The model under review builds one solid part; all positions refer to its coordinate system, in mm. Face numbers are marked on the shaded views. A direction names the side the tool comes from. Give positions to 0.01 mm unless a question says otherwise; leave off trailing zeros. Loops run counter-clockwise (first coordinate to the right, second up) from the corner with the lowest first, then second, coordinate; pieces in that order, holes last. Notation, with made-up numbers: M 11.5,86.25 L 54.5,86.25 A33 cw 54.5,125.25 Z; hole C 46.5,-26 d9. An arc over 180 degrees is marked long. Return JSON: item names as keys, results as strings. Group by question number.
```python
from build123d import *

# Parameters (mm, degrees)
EXTRUDE_1_DEPTH     = 35
EXTRUDE_2_DEPTH     = 3
SKETCH_3_R          = 4
CUT_EXTRUDE_1_DEPTH = 112.130553854
SKETCH_4_R          = 4
CUT_EXTRUDE_2_DEPTH = 112.130553854
FILLET_1_R          = 2
FILLET_2_R          = 2


with BuildPart() as part:
    # 草图1 → 凸台-拉伸1 (new body)
    with BuildSketch(Plane.XY):
        Polygon((0, 0), (78, 0), (78, 78), (71, 78), (71, 7), (0, 7), align=None)
    extrude(amount=EXTRUDE_1_DEPTH)

    # 草图2 → 凸台-拉伸2 (add)
    with BuildSketch(Plane(origin=(0, 0, 0), x_dir=(-1, 0, 0), z_dir=(0, 0, -1))):
        Polygon((-78, 78), (-78, 0), (0, 0), (0, 12.5), (-8, 12.5), (-65.5, 70), (-65.5, 78), align=None)
    extrude(amount=EXTRUDE_2_DEPTH)

    # 草图3 → 切除-拉伸1 (cut, through all)
    with BuildSketch(Plane.ZY.offset(-71)):
        with Locations((16, 58)):
            Circle(SKETCH_3_R)
        with BuildLine():
            Line((12, 41), (12, 23))
            ThreePointArc((12, 23), (16, 19), (20, 23))
            Line((20, 23), (20, 41))
            ThreePointArc((20, 41), (16, 45), (12, 41))
        make_face()
    extrude(amount=-CUT_EXTRUDE_1_DEPTH, mode=Mode.SUBTRACT)

    # 草图4 → 切除-拉伸2 (cut, through all)
    with BuildSketch(Plane(origin=(0, 7, 0), x_dir=(1, 0, 0), z_dir=(0, 1, 0))):
        with Locations(Location((20, -16, 0), (0, 0, 270))):
            Circle(SKETCH_4_R)
        with BuildLine():
            Line((37, -20), (55, -20))
            ThreePointArc((55, -20), (59, -16), (55, -12))
            Line((55, -12), (37, -12))
            ThreePointArc((37, -12), (33, -16), (37, -20))
        make_face()
    extrude(amount=-CUT_EXTRUDE_2_DEPTH, mode=Mode.SUBTRACT)

    # 圆角1
    fillet_1_edges = [part.edges().sort_by_distance(p)[0] for p in [
        (65.5, 78, -1.5),
        (0, 12.5, -1.5),
    ]]
    fillet(fillet_1_edges, radius=FILLET_1_R)

    # 圆角2
    fillet_2_edges = [part.edges().sort_by_distance(p)[0] for p in [
        (8, 12.5, -1.5),
        (65.5, 70, -1.5),
    ]]
    fillet(fillet_2_edges, radius=FILLET_2_R)


solid = part.part
```
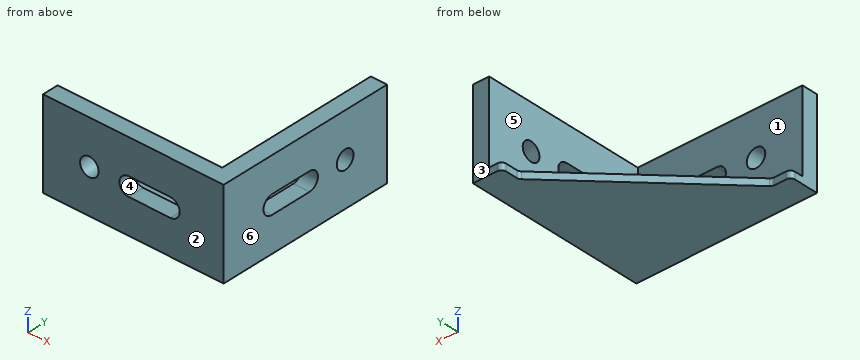
(1) For probe 1 along X at (y, z) = (4.25, 16); probe 2 along Y at (x, z) = (73.75, 16); probe 3 along Y at (x, z) = (62, 7), list the stretches that pass through material, from the lowest coordinate up.
(2) Add section D-D (x = 73). Write out the cut boundary in (y, z).
(3) For the marked faces 1 and 2, list the 3-axis set-ups (+Z, -Z, +X, -X, +Y, -Y) from which the entire face can be reached by the end or side of a thin tool; tool diameter is ignored.
(4) For pin 1 (4 mm diameter, centred on x = 19.5, z = 9.5, fed in from +Y); pin 2 (4 mm diameter, centred on y = 13.5, z = 19, fed in from -X); pin 3 (3.5 mm diameter, centred on x = 5, z = -1.5, fed in from +Y), all flat-tipped, find the tip position at first contact; note any pin that passes through.
(5) Mouldability with a two-part tool opening along X and no side actions: class the marked faces 3, 4, 5 and 6 as released by +X, released by -X, zero draft, split by the parting line, or undercut.
(6) Add section B-B (z = 16). Write out the cut boundary in (x, y), and give its area (3 significant figures).
(7) Add section A-A (x = 52.5). Write out the cut boundary in (y, z).
(8) Add section C-C (y = 38). Write out the cut boundary in (x, z).
Verdict:
{
 "1": {"probe 1": "x = 0 to 16, 24 to 33, 59 to 78", "probe 2": "y = 0 to 19, 45 to 54, 62 to 78", "probe 3": "y = 0 to 7"},
 "2": {"outline": "M 0,-3 L 78,-3 L 78,35 L 0,35 Z; hole M 23,12 L 41,12 A4 ccw 41,20 L 23,20 A4 ccw Z; hole C 58,16 d8"},
 "3": {"face 1": "+Z, -X, +Y", "face 2": "+Z, -Z, +X, -X, -Y"},
 "4": {"pin 1": "stops at y = 7", "pin 2": "stops at x = 71", "pin 3": "stops at y = 12.5"},
 "5": {"face 3": "zero draft", "face 4": "undercut", "face 5": "released by -X", "face 6": "released by +X"},
 "6": {"outline": "M 0,0 L 16,0 L 16,7 L 0,7 Z; M 24,0 L 33,0 L 33,7 L 24,7 Z; M 59,0 L 78,0 L 78,19 L 71,19 L 71,7 L 59,7 Z; M 71,45 L 78,45 L 78,54 L 71,54 Z; M 71,62 L 78,62 L 78,78 L 71,78 Z", "area": "567 mm²"},
 "7": {"outline": "M 0,-3 L 57,-3 L 57,0 L 7,0 L 7,12 L 0,12 Z; M 0,20 L 7,20 L 7,35 L 0,35 Z"},
 "8": {"outline": "M 33.5,-3 L 78,-3 L 78,12 L 71,12 L 71,0 L 33.5,0 Z; M 71,20 L 78,20 L 78,35 L 71,35 Z"}
}
